```python
from build123d import *

# Parameters (mm, degrees)
RESSALTO_EXTRUS_O1_DEPTH = 20
ESBO_O2_R                = 2.5
CORTE_EXTRUS_O2_DEPTH    = 2


with BuildPart() as part:
    # Esboço1 → Ressalto-extrusão1 (new body)
    with BuildSketch(Plane.XY):
        with BuildLine():
            Line((191.678372413, 42.279236252), (191.678372413, -7.720763748))
            ThreePointArc((191.678372413, -7.720763748), (141.678372413, -57.720763748), (91.678372413, -7.720763748))
            Line((91.678372413, -7.720763748), (91.678372413, 42.279236252))
            Line((91.678372413, 42.279236252), (61.678372413, 42.279236252))
            Line((61.678372413, 42.279236252), (61.678372413, 40.779236252))
            Line((61.678372413, 40.779236252), (90.178372413, 40.779236252))
            Line((90.178372413, 40.779236252), (90.178372413, -7.720763748))
            ThreePointArc((90.178372413, -7.720763748), (141.678372413, -59.220763748), (193.178372413, -7.720763748))
            Line((193.178372413, -7.720763748), (193.178372413, 40.779236252))
            Line((193.178372413, 40.779236252), (221.678372413, 40.779236252))
            Line((221.678372413, 40.779236252), (221.678372413, 42.279236252))
            Line((221.678372413, 42.279236252), (191.678372413, 42.279236252))
        make_face()
    extrude(amount=RESSALTO_EXTRUS_O1_DEPTH)

    # Esboço2 → Corte-extrusão2 (cut)
    with BuildSketch(Plane.XZ.offset(-40.779236252)):
        with Locations(Location((75.928372413, 10, 0), (0, 0, 270))):
            Circle(ESBO_O2_R)
        with Locations(Location((207.428372413, 10, 0), (0, 0, 270))):
            Circle(ESBO_O2_R)
    extrude(amount=-CORTE_EXTRUS_O2_DEPTH, mode=Mode.SUBTRACT)


solid = part.part
```
Read the model definition and answer for the solid it produces. Units are mm, in the model's axes. A direction names the side the tool comes from. Give positions to 0.01 mm unless a question says otherwise; leave off trailing zeros. Write each loop counter-clockwise with the first axis right and the second up, starting at its lowest first coordinate (ties: lowest second). Pieces come first, ordered by that corner, then holes. Notation, with made-up numbers: M 38.5,29.5 L 52.5,29.5 A32 cw 52.5,59.5 Z; hole C 25,38 d8. An arc over 180 degrees is marked long. Put each result on its own line as item: value. Start each with the question number.
1. The part is cut by section C-C, the plane y = -25. Give the vertices of the cut face in (x, z), and give its area (3 significant figures).
2. The part is cut by section A-A, the plane y = 8. Give the vertices of the cut face in (x, z), and give its area (3 significant figures).
3. The part is cut by section B-B, the plane z = 10. Give the vertices of the cut face in (x, y).
4. Each of these flat-tipped pins is pushed along its axis until it touches: pin 1 Ø3 at (x, z) = (159.5, 7) entering from -Y; pin 2 Ø10 at (x, z) = (118.5, 16) entering from +Y; pin 3 Ø10 at (y, z) = (5.5, 13.5) entering from -X. Where does it stop, or does it pass through?
5. Which of the six approach directions +Z, -Z, +X, -X, +Y, -Y give full straight-line access (tool end or side, diameter ignored) to faces 1 (the flat face through (80, 42.279, 10)), 2 (the flat face through (191.678, 18, 10)), 3 (the flat face through (79, 40.779, 10))?
6. Consider line 1 along X through (y, z) = (41.4, 10); line 2 along X through (y, z) = (21.5, 6.75); line 3 along X through (y, z) = (-9.5, 10.75). Determine where each line is inside the solid, lowest interval first.
7. For a pull along X with two mould halves and no side action, classify faces 4 (the flat face through (90.178, 17, 10)), 5 (the flat face through (210.4, 40.779, 9.9)), 6 (the cylindrical face through (142.78, -57.71, 9.86)), 7 (the flat face through (193.178, 16, 10)) as released by +X, released by -X, zero draft, split by the parting line, or undercut.
8. The part is cut by section D-D, the plane x = 83. Give the vertices of the cut face in (y, z).
Final values:
1. outline: M 93.16,0 L 94.76,0 L 94.76,20 L 93.16,20 Z; M 188.6,0 L 190.19,0 L 190.19,20 L 188.6,20 Z
1. area: 63.8 mm²
2. outline: M 90.18,0 L 91.68,0 L 91.68,20 L 90.18,20 Z; M 191.68,0 L 193.18,0 L 193.18,20 L 191.68,20 Z
2. area: 60.0 mm²
3. outline: M 61.68,40.78 L 73.43,40.78 L 73.43,42.28 L 61.68,42.28 Z; M 78.43,40.78 L 90.18,40.78 L 90.18,-7.72 A51.5 ccw 193.18,-7.72 L 193.18,40.78 L 204.93,40.78 L 204.93,42.28 L 191.68,42.28 L 191.68,-7.72 A50 cw 91.68,-7.72 L 91.68,42.28 L 78.43,42.28 Z; M 209.93,40.78 L 221.68,40.78 L 221.68,42.28 L 209.93,42.28 Z
4. pin 1: stops at y = -56.57
4. pin 2: stops at y = -49.02
4. pin 3: stops at x = 90.18
5. face 1: +Z, -Z, +X, -X, +Y
5. face 2: +Z, -Z, +Y
5. face 3: +Z, -Z, -X, -Y
6. line 1: x = 61.68 to 73.43, 78.43 to 91.68, 191.68 to 204.93, 209.93 to 221.68
6. line 2: x = 90.18 to 91.68, 191.68 to 193.18
6. line 3: x = 90.21 to 91.71, 191.65 to 193.15
7. face 4: released by -X
7. face 5: zero draft
7. face 6: undercut
7. face 7: released by +X
8. outline: M 40.78,0 L 42.28,0 L 42.28,20 L 40.78,20 Z
